```python
from build123d import *

# Parameters (mm, degrees)
BOSS_EXTRUDE1_DEPTH   = 5
SKETCH2_R             = 4.5
CUT_EXTRUDE1_DEPTH    = 4
SKETCH7_R             = 3
CUT_EXTRUDE3_DEPTH    = 0.5
BODY_MOVE_COPY1_ANGLE = 90
BODY_MOVE_COPY2_ANGLE = 180
SKETCH8_R             = 2.5
BOSS_EXTRUDE2_DEPTH   = 5
CUT_EXTRUDE4_START    = -4
SKETCH9_R             = 2.5
SKETCH9_R_2           = 2
CUT_EXTRUDE4_DEPTH    = 4


with BuildPart() as part:
    # Sketch1 → Boss-Extrude1 (new body)
    with BuildSketch(Plane.XY):
        with BuildLine():
            Line((0.638194143, 7.974499314), (100.159744623, 3.998531964))
            ThreePointArc((100.159744623, 3.998531964), (104.001721656, 0), (100.159744623, -3.998531964))
            Line((100.159744623, -3.998531964), (0.638194143, -7.974499314))
            ThreePointArc((0.638194143, -7.974499314), (-7.999995692, 0), (0.638194143, 7.974499314))
        make_face()
    extrude(amount=BOSS_EXTRUDE1_DEPTH)

    # Sketch2 → Cut-Extrude1 (cut)
    with BuildSketch(Plane(origin=(0, 0, 0), x_dir=(-1, 0, 0), z_dir=(0, 0, -1))):
        Circle(SKETCH2_R)
    extrude(amount=-CUT_EXTRUDE1_DEPTH, mode=Mode.SUBTRACT)

    # Sketch7 → Cut-Extrude3 (cut)
    with BuildSketch(Plane(origin=(0, 0, 4), x_dir=(-1, 0, 0), z_dir=(0, 0, -1))):
        Circle(SKETCH7_R)
    extrude(amount=-CUT_EXTRUDE3_DEPTH, mode=Mode.SUBTRACT)


with BuildPart() as part_1:
    # Body-Move_Copy1: moved
    add(part.part.rotate(Axis((0, 0, 11), (-1, 0, 0)), BODY_MOVE_COPY1_ANGLE))


with BuildPart() as part_2:
    # Body-Move_Copy2: moved
    add(part_1.part.rotate(Axis((0, -8, 11), (1, 0, 0)), BODY_MOVE_COPY2_ANGLE))

    # Sketch8 → Boss-Extrude2 (add)
    with BuildSketch(Plane.XZ.offset(10)):
        with Locations(Location((100, 11, 0), (0, 0, 270))):
            Circle(SKETCH8_R)
    extrude(amount=BOSS_EXTRUDE2_DEPTH)

    # Sketch9 → Cut-Extrude4 (cut)
    with BuildSketch(Plane.XZ.offset(15).offset(CUT_EXTRUDE4_START)):
        with Locations(Location((100, 11, 0), (0, 0, 270))):
            Circle(SKETCH9_R)
        with Locations(Location((100, 11, 0), (0, 0, 270))):
            Circle(SKETCH9_R_2, mode=Mode.SUBTRACT)
    extrude(amount=CUT_EXTRUDE4_DEPTH, mode=Mode.SUBTRACT)


solid = part_2.part
```
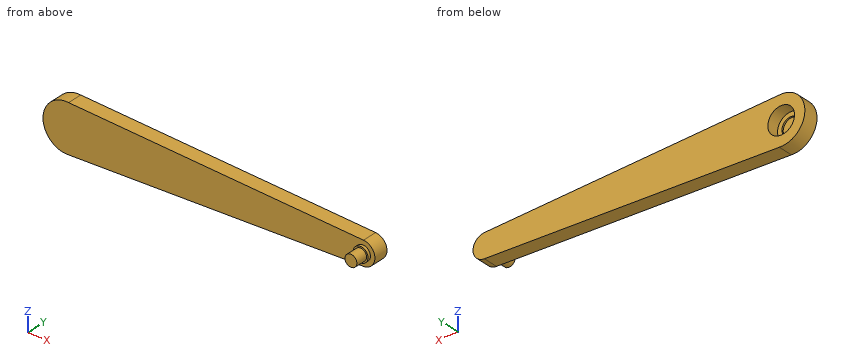
Could you check a few things on this model? Use its own coordinates, in mm. Round coordinates to 2 decimals unless told otherwise and drop trailing zeros. Loops run counter-clockwise (first coordinate to the right, second up) from the corner with the lowest first, then second, coordinate; pieces in that order, holes last. Notation, with made-up numbers: M 24.25,36.5 L 51.25,36.5 A22 cw 51.25,57.5 Z; hole C 55.5,25.25 d4. An arc over 180 degrees is marked long. Put each result on its own line as item: value.
Q1. Imagine slicing it at B-B (z = 11). Write out the boundary of the cut face in (x, y), then the cut area to 3 significant figures.
Check result:
outline: M -8,-10 L 97.5,-10 L 97.5,-11 L 98,-11 L 98,-15 L 102,-15 L 102,-11 L 102.5,-11 L 102.5,-10 L 104,-10 L 104,-5 L 4.5,-5 L 4.5,-9 L 3,-9 L 3,-9.5 L -3,-9.5 L -3,-9 L -4.5,-9 L -4.5,-5 L -8,-5 Z
area: 542 mm2
Q2. Imagine slicing it at A-A (y = -7.75). Write out the boundary of the cut face in (x, z), then the cut area to 3 significant figures.
Check result:
outline: M 0.64,3.03 L 100.16,7 A4 ccw 100.16,15 L 0.64,18.97 A8 ccw long Z; hole C 0,11 d9
area: 1,260 mm2
Q3. Imagine slicing it at D-D (x = 7.5). Write out the boundary of the cut face in (y, z).
Check result:
outline: M -10,3.3 L -5,3.3 L -5,18.7 L -10,18.7 Z
Q4. I need wall thicknesses on probe 1 along Z at (x, y) = (0, -9.35); probe 2 along Z at (x, y) = (0, -8); probe 3 along Y at (x, z) = (88, 7.75). Which ranges of each line are inside material? Lowest first, please.
Check result:
probe 1: 3 to 8, 14 to 19
probe 2: 3 to 6.5, 15.5 to 19
probe 3: -10 to -5
Q5. Imagine slicing it at C-C (y = -14). Write out the boundary of the cut face in (x, z).
Check result:
outline: C 100,11 d4
Q6. For pin 1 (1.5 mm diameter, centred on y = -6, z = 6, fed in from -X); pin 2 (8 mm diameter, centred on x = 0, z = 11, fed in from +Y); pin 3 (8 mm diameter, centred on x = 26, z = 10, fed in from -Y), each with a flat end and sliding along its axis, tell me the tip position at first contact or that it passes through.
Check result:
pin 1: x = -6.78
pin 2: y = -9
pin 3: y = -10
